from build123d import *

# Parameters (mm, degrees)
ESBO_O1_R                = 2
RESSALTO_EXTRUS_O2_DEPTH = 2


with BuildPart() as part:
    # Esboço1 → Ressalto-extrusão2 (new body)
    with BuildSketch(Plane.XY):
        Polygon((-0.066609968, -5.044992778), (0.066609968, -5.044992778), (21.752134594, -5.044992778), (31.476547475, -29.544992778), (69.476547475, -29.544992778), (69.476547475, -17.544992778), (35.678254574, -17.544992778), (22.778523201, 14.955007222), (-22.778523201, 14.955007222), (-35.678254574, -17.544992778), (-69.476547475, -17.544992778), (-69.476547475, -29.544992778), (-31.476547475, -29.544992778), (-21.752134594, -5.044992778), align=None)
        with Locations((-63.476547475, -23.544992778)):
            Circle(ESBO_O1_R, mode=Mode.SUBTRACT)
        with Locations((-37.476547475, -23.544992778)):
            Circle(ESBO_O1_R, mode=Mode.SUBTRACT)
        with Locations((37.476547475, -23.544992778)):
            Circle(ESBO_O1_R, mode=Mode.SUBTRACT)
        with Locations((63.476547475, -23.544992778)):
            Circle(ESBO_O1_R, mode=Mode.SUBTRACT)
    extrude(amount=RESSALTO_EXTRUS_O2_DEPTH)


solid = part.part
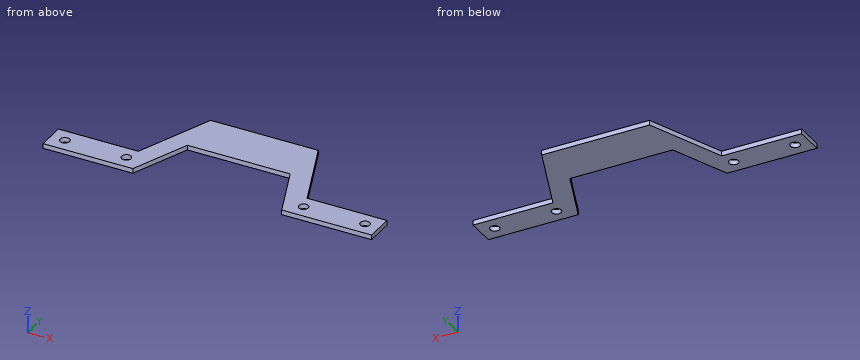
Read the model definition and answer for the solid it produces. Units are mm, in the model's axes. Round coordinates to 2 decimals unless told otherwise and drop trailing zeros. Loops run counter-clockwise (first coordinate to the right, second up) from the corner with the lowest first, then second, coordinate; pieces in that order, holes last.
Q1. Section B-B on y = -12.5 is taken. Write down the section's boundary in (x, z), and give its area (3 significant figures).
Q2. Consider probe 1 along Y at (x, z) = (4, 0.7) (3 decimals); probe 2 along X at (y, z) = (-25, 0.65); probe 3 along Y at (x, z) = (-59.5, 1.7) (3 decimals). Determine where each line is inside the solid, lowest interval first.
Q3. Section A-A on z = 1.1 is taken. Write down the section's boundary in (x, y) (3 decimals).
Q4. Section D-D on y = 9 is taken. Write down the section's boundary in (x, z).
Q5. Each of these flat-tipped pins is pushed along its axis until it touches: pin 1 (6.5 mm diameter, centred on x = -37.48, y = -23.54, fed in from +Z); pin 2 (5 mm diameter, centred on x = 34.5, y = -6, fed in from +Z). Where does it stop, or does it pass through?
Q6. Section C-C on x = -59 is taken. Write down the section's boundary in (y, z) (3 decimals), and give its area (3 significant figures).
Output:
1. outline: (-33.68, 0) - (-24.71, 0) - (-24.71, 2) - (-33.68, 2) - close; (24.71, 0) - (33.68, 0) - (33.68, 2) - (24.71, 2) - close
1. area: 35.9 mm2
2. probe 1: y = -5.045 to 14.955
2. probe 2: x = -69.48 to -64.85, -62.1 to -38.85, -36.1 to -29.67, 29.67 to 36.1, 38.85 to 62.1, 64.85 to 69.48
2. probe 3: y = -29.545 to -17.545
3. outline: (-69.477, -29.545) - (-31.477, -29.545) - (-21.752, -5.045) - (21.752, -5.045) - (31.477, -29.545) - (69.477, -29.545) - (69.477, -17.545) - (35.678, -17.545) - (22.779, 14.955) - (-22.779, 14.955) - (-35.678, -17.545) - (-69.477, -17.545) - close; hole circle Ø4 at (-63.477, -23.545); hole circle Ø4 at (-37.477, -23.545); hole circle Ø4 at (37.477, -23.545); hole circle Ø4 at (63.477, -23.545)
4. outline: (-25.14, 0) - (25.14, 0) - (25.14, 2) - (-25.14, 2) - close
5. pin 1: stops at z = 2
5. pin 2: passes through
6. outline: (-29.545, 0) - (-17.545, 0) - (-17.545, 2) - (-29.545, 2) - close
6. area: 24.0 mm2
